Source: CAD feature listing. Evaluate the final solid. Frame: model axes, mm. Face numbers are marked on the shaded views. A direction names the side the tool comes from. Coordinates: 2 decimals unless noted, no trailing zeros. Order: outer loops, then holes, each group sorted by start corner. A loop starts at its lowest first (then second) coordinate and runs counter-clockwise, first axis right, second up.
```python
from build123d import *

# Parameters (mm, degrees)
EXTRUDE_1_DEPTH     = 19
FILLET_1_R          = 1
SKETCH_2_R          = 1
CUT_EXTRUDE_1_DEPTH = 500000
FILLET_2_R          = 5
FILLET_3_R          = 5
SKETCH_3_R          = 3.05
SKETCH_3_R_2        = 1.5
CUT_EXTRUDE_2_DEPTH = 500


with BuildPart() as part:
    # 草图1 → 凸台-拉伸1 (new body)
    with BuildSketch(Plane(origin=(0, 0, 0), x_dir=(0, 0, -1), z_dir=(1, 0, 0))):
        Polygon((-20, -12.94), (-20, 10.94), (20, 10.94), (20, -12.94), (22, -12.94), (22, 12.94), (-22, 12.94), (-22, -12.94), align=None)
    extrude(amount=EXTRUDE_1_DEPTH)

    # 圆角1
    fillet_1_edges = [part.edges().sort_by_distance(p)[0] for p in [
        (9.5, 10.94, -20),
        (9.5, 10.94, 20),
        (9.5, 12.94, 22),
        (9.5, 12.94, -22),
    ]]
    fillet(fillet_1_edges, radius=FILLET_1_R)

    # 草图2 → 切除-拉伸1 (cut)
    with BuildSketch(Plane.XY.offset(22)):
        with Locations((2.5, -3.56)):
            Circle(SKETCH_2_R)
        with Locations((16.5, -3.56)):
            Circle(SKETCH_2_R)
        with Locations((9.5, -10.56)):
            Circle(SKETCH_2_R)
        with Locations((9.5, 3.44)):
            Circle(SKETCH_2_R)
    extrude(amount=-CUT_EXTRUDE_1_DEPTH, mode=Mode.SUBTRACT)

    # 圆角2
    fillet_2_edges = [part.edges().sort_by_distance(p)[0] for p in [
        (19, -12.94, 21),
        (0, -12.94, 21),
    ]]
    fillet(fillet_2_edges, radius=FILLET_2_R)

    # 圆角3
    fillet_3_edges = [part.edges().sort_by_distance(p)[0] for p in [
        (0, -12.94, -21),
        (19, -12.94, -21),
    ]]
    fillet(fillet_3_edges, radius=FILLET_3_R)

    # 草图3 → 切除-拉伸2 (cut)
    with BuildSketch(Plane(origin=(0, 12.94, 0), x_dir=(1, 0, 0), z_dir=(0, 1, 0))):
        with Locations(Location((9.5, 0, 0), (0, 0, 270))):
            Circle(SKETCH_3_R)
        with Locations(Location((4.5, 5, 0), (0, 0, 270))):
            Circle(SKETCH_3_R_2)
        with Locations(Location((14.5, 5, 0), (0, 0, 270))):
            Circle(SKETCH_3_R_2)
        with Locations(Location((14.5, -5, 0), (0, 0, 270))):
            Circle(SKETCH_3_R_2)
        with Locations(Location((4.5, -5, 0), (0, 0, 270))):
            Circle(SKETCH_3_R_2)
    extrude(amount=-CUT_EXTRUDE_2_DEPTH, mode=Mode.SUBTRACT)


solid = part.part
```
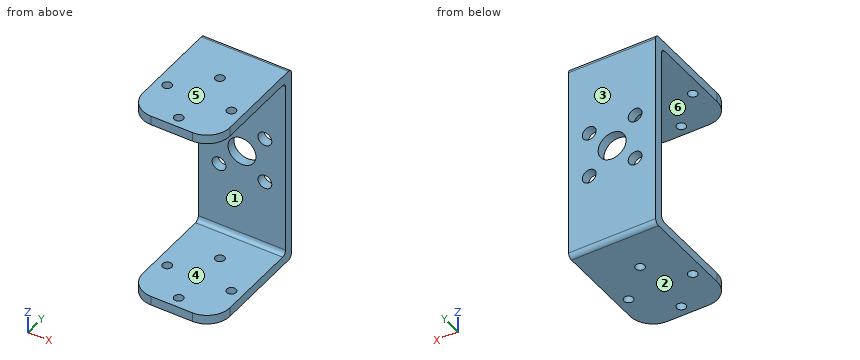
1. Ray query, line 1 (X direction, y = 11.55, z = -5); line 2 (Y direction, x = 9.5, z = 20.8); line 3 (Z direction, x = 14.25, y = -3.75). Return the intervals inside material, ascending.
Findings:
line 1: x = 0 to 3, 6 to 13, 16 to 19
line 2: y = -12.94 to -11.56, -9.56 to 2.44, 4.44 to 12.94
line 3: z = -22 to -20, 20 to 22
2. Section query D-D on y = 0.5. Return loops of the section in (x, z), plus the area to 3 significant figures.
Findings:
outline: (0, -22) - (19, -22) - (19, -20) - (0, -20) - close; (0, 20) - (19, 20) - (19, 22) - (0, 22) - close
area: 76.0 mm2
3. Draft query along Z for the marked faces 1, 2, 3 and 4. Return one class per face: released by +Z, released by -Z, zero draft, split by the parting line, or undercut.
Findings:
face 1: undercut
face 2: released by -Z
face 3: zero draft
face 4: undercut
4. Access query for the marked faces 5 and 6. Directions: +Z, -Z, +X, -X, +Y, -Y. A direction counts if a zero-diameter tool reaches every point of the face in a straight line with its end or side. Return the directions, or none.
Findings:
face 5: +Z, +X, -X, +Y, -Y
face 6: +X, -X, -Y
5. Section query C-C on y = 3.44. Return loops of the section in (x, z), plus the area to 3 significant figures.
Findings:
outline: (0, -22) - (8.5, -22) - (8.5, -20) - (0, -20) - close; (0, 20) - (8.5, 20) - (8.5, 22) - (0, 22) - close; (10.5, -22) - (19, -22) - (19, -20) - (10.5, -20) - close; (10.5, 20) - (19, 20) - (19, 22) - (10.5, 22) - close
area: 68.0 mm2
6. Section query A-A on z = 0. Return loops of the section in (x, y).
Findings:
outline: (0, 10.94) - (6.45, 10.94) - (6.45, 12.94) - (0, 12.94) - close; (12.55, 10.94) - (19, 10.94) - (19, 12.94) - (12.55, 12.94) - close
7. Section query B-B on x = 9.5. Count the separate pieces of the cut face and the enclosed holes in it, plus the area to 3 significant figures.
Findings:
separate pieces: 6
enclosed holes: 0
area: 155 mm2
8. Pin query (flat end, axial travel): P1, Ø5.5, axis at x = 7.5, z = 1, coming from the -Y side. Return the tip coordinate at first contact, or that it passes through.
Findings:
P1: stops at y = 10.94
